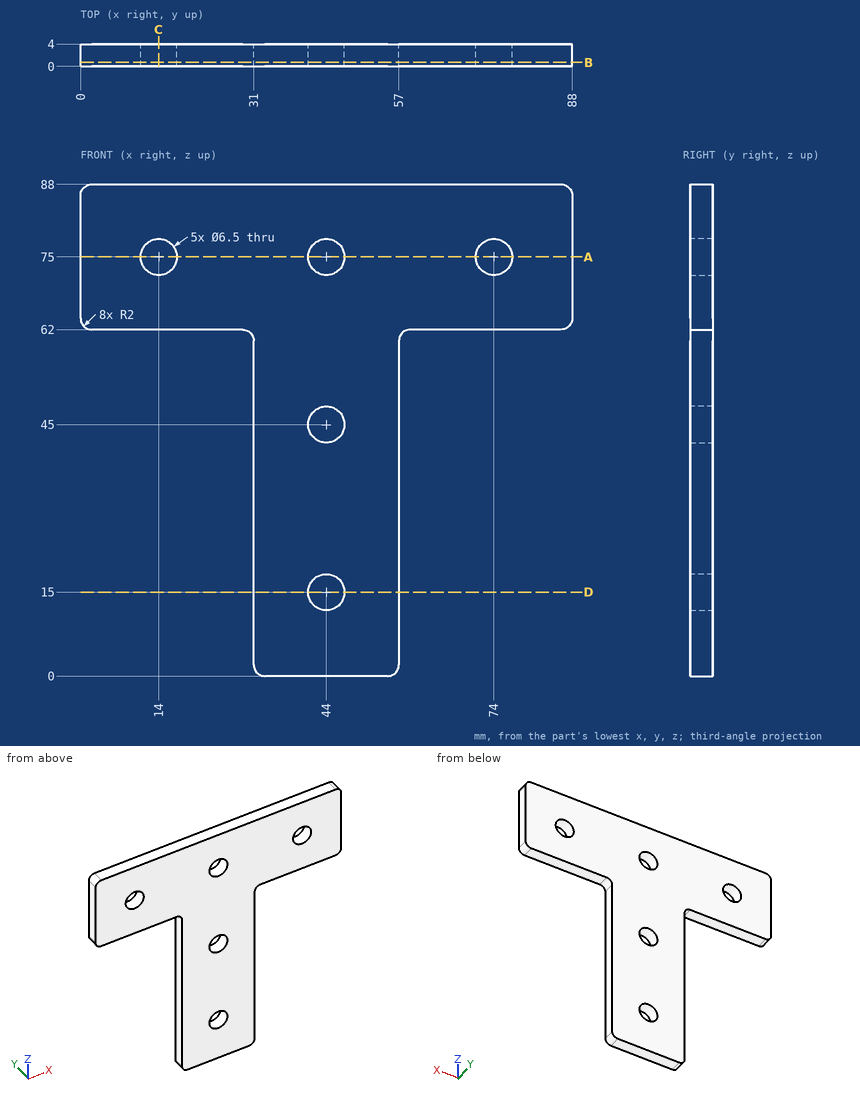
Job drawing, mm, ordinate dimensions from the low corner. One solid piece. Coordinates: 2 decimals unless noted, no trailing zeros. Order: outer loops, then holes, each group sorted by start corner. A loop starts at its lowest first (then second) coordinate and runs counter-clockwise, first axis right, second up. Notation, with made-up numbers: (65, 29) - (88, 29) arc R16 ccw to (88, 36) - close; hole circle Ø7 at (37.5, -19). An arc over 180 degrees is marked (long way). Write each question's results on one line, items separated by ' | '. Start each with the question number.
Item 1: Band-saw the part on C-C on x = 14. Write the cut outline in (y, z).
Item 2: Flat gauge pins, fed straight in: pin 1 (1.2 mm diameter, centred on x = 78, y = 1.5, fed in from -Z); pin 2 (1 mm diameter, centred on y = 3.5, z = 57, fed in from -X); pin 3 (4 mm diameter, centred on x = 44, z = 45, fed in from +Y); pin 4 (1.2 mm diameter, centred on y = 1, z = 40.5, fed in from +X). Where does each tip first touch, or does it go through?
Item 3: Band-saw the part on D-D on z = 15. Write the cut outline in (x, y), and give its area (3 significant figures).
Item 4: Band-saw the part on A-A on z = 75. Write the cut outline in (x, y).
Item 5: Wall check: probe 1 along X at (y, z) = (3, 75); probe 2 along X at (y, z) = (1.25, 15); probe 3 along X at (y, z) = (3.2, 11). Give the ranges that are in metal, low to high. Write a range as [from, to].
Item 6: Band-saw the part on B-B on y = 0.7. Write the cut outline in (x, z).
Numbers:
1) outline: (0, 62) - (4, 62) - (4, 71.75) - (0, 71.75) - close; (0, 78.25) - (4, 78.25) - (4, 88) - (0, 88) - close
2) pin 1: z = 62 | pin 2: x = 31 | pin 3: through | pin 4: x = 57
3) outline: (31, 0) - (40.75, 0) - (40.75, 4) - (31, 4) - close; (47.25, 0) - (57, 0) - (57, 4) - (47.25, 4) - close | area: 78.0 mm^2
4) outline: (0, 0) - (10.75, 0) - (10.75, 4) - (0, 4) - close; (17.25, 0) - (40.75, 0) - (40.75, 4) - (17.25, 4) - close; (47.25, 0) - (70.75, 0) - (70.75, 4) - (47.25, 4) - close; (77.25, 0) - (88, 0) - (88, 4) - (77.25, 4) - close
5) probe 1: [0, 10.75], [17.25, 40.75], [47.25, 70.75], [77.25, 88] | probe 2: [31, 40.75], [47.25, 57] | probe 3: [31, 57]
6) outline: (0, 64) arc R2 ccw to (2, 62) - (29, 62) arc R2 cw to (31, 60) - (31, 2) arc R2 ccw to (33, 0) - (55, 0) arc R2 ccw to (57, 2) - (57, 60) arc R2 cw to (59, 62) - (86, 62) arc R2 ccw to (88, 64) - (88, 86) arc R2 ccw to (86, 88) - (2, 88) arc R2 ccw to (0, 86) - close; hole circle Ø6.5 at (14, 75); hole circle Ø6.5 at (44, 15); hole circle Ø6.5 at (44, 45); hole circle Ø6.5 at (44, 75); hole circle Ø6.5 at (74, 75)
